Here's how the part is built. I have some questions about the finished solid (model axes, mm). A direction names the side the tool comes from. Give positions to 0.01 mm unless a question says otherwise; leave off trailing zeros. Loops run counter-clockwise (first coordinate to the right, second up) from the corner with the lowest first, then second, coordinate; pieces in that order, holes last. Notation, with made-up numbers: M 64.5,6 L 69.5,6 A25 cw 69.5,44 Z; hole C 49,10 d10. An arc over 180 degrees is marked long. Answer as CSV lines item,"result". Start each with the question number.
Item 1: Will these pins go through, and if not, where does the flat tip stop? P1, Ø6, axis at x = 68.5, y = 7.5, coming from the +Z side; P2, Ø6, axis at y = 21.5, z = 4.5, coming from the -X side; P3, Ø2.5, axis at x = 6.5, z = 6.5, coming from the +Y side.
Item 2: I want a section at C-C on y = 5.5. List the corners of the cut face in (x, z) for me.
Item 3: If we mould it in two halves opening along Y, with no side actions, what happens to faces 3 (the flat face through (36, 0, 5)), 4 (the flat face through (0, 6, 5)), 5 (the flat face through (37, 24, 6)), 6 (the flat face through (31, 30, 6))? For each: released by +Y, released by -Y, zero draft, split by the parting line, or undercut.
Item 4: For faces 1 (the flat face through (43, 30, 6)), 2 (the flat face through (36, 15, 0)), which set-ups out of +Z, -Z, +X, -X, +Y, -Y let a thin tool reach every point of the face, with its end or its side?
Item 5: I want a section at D-D on x = 20. List the corners of the cut face in (y, z) for me.
Item 6: I want a section at B-B on y = 28.5. List the corners of the cut face in (x, z) for me, plus the area to 3 significant figures.
Item 7: I want a section at A-A on x = 36. List the corners of the cut face in (y, z) for me.
Item 8: If I drill on line 1 along X through (y, z) = (7, 7); line 2 along Y through (x, z) = (40.5, 3); line 3 along X through (y, z) = (34, 5.25), over which ranges is the centre line in solid material (lowest first)? Write a range as from..to.
Autodesk Fusion 360 part; units mm, degrees
sketch "Sketch1" plane through (0, 0, 0) normal (0, 0, 1) x (1, 0, 0)
  line L0 (0, 0) -> (74, 0)
  line L1 (0, 0) -> (0, 13)
  line L2 (37, 0) -> (37, 38) construction
  line L3 (37, 38) -> (27, 38)
  line L4 (0, 13) -> (27, 38)
  line L5 (37, 38) -> (47, 38)
  line L6 (74, 0) -> (74, 13)
  line L7 (74, 13) -> (47, 38)
  dimension "d1" = 74
  dimension "d2" = 13
  dimension "d3" = 38
  dimension "d4" = 10
  dimension "d5" = 10
  dimension "d6" = 13
extrude "Extrude1" add sketch "Sketch1" along normal blind 10
sketch "Sketch2" plane through (0, 0, 10) normal (0, 0, 1) x (-1, 0, 0)
  line L0 (0, 0) -> (-74, 0)
  line L1 (-74, 0) -> (-74, -13)
  line L2 (-74, -13) -> (-47, -38)
  line L3 (-47, -38) -> (-27, -38)
  line L4 (-27, -38) -> (0, -13)
  line L5 (0, -13) -> (0, 0)
  line L6 (-37, -36) -> (-31, -36) construction
  line L7 (0, 0) -> (-2, 0) construction
  line L8 (-2, 0) -> (-2, -2) construction
  line L9 (-74, 0) -> (-72, 0) construction
  line L10 (-72, 0) -> (-72, -2) construction
  line L11 (-31, -36) -> (-43, -36)
  line L12 (-43, -36) -> (-43, -24)
  line L13 (-43, -24) -> (-31, -24)
  line L14 (-31, -24) -> (-31, -36)
  line L15 (-2, -2) -> (-14, -2)
  line L16 (-14, -2) -> (-14, -14)
  line L17 (-14, -14) -> (-2, -14)
  line L18 (-2, -14) -> (-2, -2)
  line L19 (-72, -2) -> (-60, -2)
  line L20 (-60, -2) -> (-60, -14)
  line L21 (-60, -14) -> (-72, -14)
  line L22 (-72, -14) -> (-72, -2)
  dimension "d10" = 6
  dimension "d11" = 2
  dimension "d12" = 2
  dimension "d13" = 2
  dimension "d14" = 2
  dimension "d15" = 12
  dimension "d16" = 12
  dimension "d17" = 12
  dimension "d18" = 12
  dimension "d19" = 12
  dimension "d20" = 12
extrude "Extrude2" cut sketch "Sketch2" against normal blind 8 contours L11 L12 L13 L14 | L15 L16 L17 L18 | L19 L20 L21 L22
Result:
1,P1,"z = 2"
1,P2,"x = 5.94"
1,P3,"y = 20.18"
2,outline,"M 0,0 L 74,0 L 74,10 L 72,10 L 72,2 L 60,2 L 60,10 L 14,10 L 14,2 L 2,2 L 2,10 L 0,10 Z"
3,face 3,"released by -Y"
3,face 4,"zero draft"
3,face 5,"undercut"
3,face 6,"undercut"
4,face 1,"+Z"
4,face 2,"-Z, +X, -X, +Y, -Y"
5,outline,"M 0,0 L 31.52,0 L 31.52,10 L 0,10 Z"
6,outline,"M 16.74,0 L 57.26,0 L 57.26,10 L 43,10 L 43,2 L 31,2 L 31,10 L 16.74,10 Z"
6,area,"309 mm^2"
7,outline,"M 0,0 L 38,0 L 38,10 L 36,10 L 36,2 L 24,2 L 24,10 L 0,10 Z"
8,line 1,"0..2, 14..60, 72..74"
8,line 2,"0..24, 36..38"
8,line 3,"22.68..31, 43..51.32"
